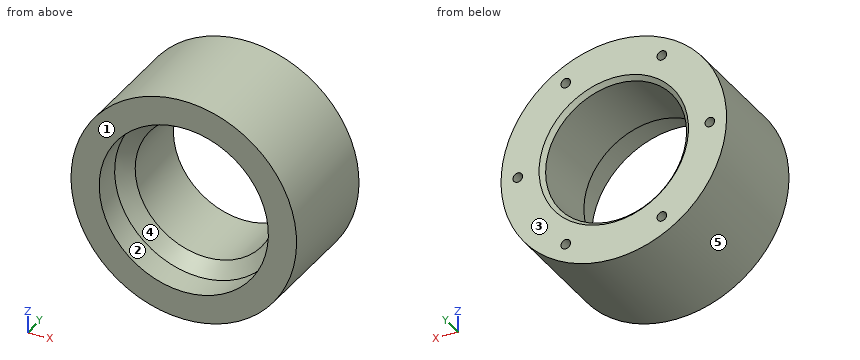
from build123d import *

# Parameters (mm, degrees)
OTW_R_GWINTOWANY_M81_D     = 6.8
OTW_R_GWINTOWANY_M81_DEPTH = 40
OTW_R_GWINTOWANY_M81_TIP   = 2.042926105


with BuildPart() as part:
    # Szkic1 → Obrót1 (revolve)
    with BuildSketch(Plane.XY, mode=Mode.PRIVATE) as obr_t1_sk:
        Polygon((-60, -4.527704194), (-60, 15.472295806), (-60, 76.472295806), (-80, 76.472295806), (-80, -4.527704194), align=None)
        Polygon((-50, 23.863292118), (-50, 73.472295806), (-53, 76.472295806), (-60, 76.472295806), (-60, 15.472295806), align=None)
    revolve(obr_t1_sk.sketch.rotate(Axis((0, 0, 0), (0, 1, 0)), 270), axis=Axis((0, 0, 0), (0, 1, 0)))

    # Otwór gwintowany M81
    with Locations(Plane(origin=(-68.136728334, 76.472295806, 0), x_dir=(0, 0, 1), z_dir=(0, 1, 0))):
        with Locations((0, 0), (-59.008137668, 34.068364167), (-59.008137668, 102.205092501), (0, 136.273456668), (59.008137668, 102.205092501), (59.008137668, 34.068364167)):
            Hole(OTW_R_GWINTOWANY_M81_D / 2, depth=OTW_R_GWINTOWANY_M81_DEPTH)
            with Locations((0, 0, -(OTW_R_GWINTOWANY_M81_DEPTH + OTW_R_GWINTOWANY_M81_TIP / 2))):  # 118° drill point
                Cone(0, OTW_R_GWINTOWANY_M81_D / 2, OTW_R_GWINTOWANY_M81_TIP, mode=Mode.SUBTRACT)


solid = part.part
Here's how the part is built. I have some questions about the finished solid (model axes, mm). Face numbers are marked on the shaded views. A direction names the side the tool comes from. Round coordinates to 2 decimals unless told otherwise and drop trailing zeros. Loops run counter-clockwise (first coordinate to the right, second up) from the corner with the lowest first, then second, coordinate; pieces in that order, holes last.
1. We'd pull the mould along Z, two halves only. Please class the marked faces 3, 4 and 5: +Z half, -Z half, draft (parallel to the pull), parting line (faces both ways), or undercut.
Answer list:
face 3: draft
face 4: undercut
face 5: parting line
2. If we section it at C-C on y = 13.5: Write out the boundary of the cut face in (x, z), plus the area to 3 significant figures.
Answer list:
outline: circle Ø160 at (0, 0); hole circle Ø120 at (0, 0)
area: 8,800 mm2
3. If we section it at B-B on y = 69.5: Write out the boundary of the cut face in (x, z).
Answer list:
outline: circle Ø160 at (0, 0); hole circle Ø6.8 at (-68.14, 0); hole circle Ø100 at (0, 0); hole circle Ø6.8 at (-34.07, -59.01); hole circle Ø6.8 at (-34.07, 59.01); hole circle Ø6.8 at (34.07, -59.01); hole circle Ø6.8 at (34.07, 59.01); hole circle Ø6.8 at (68.14, 0)
4. If I drill on line 1 along X through (y, z) = (52, 0); line 2 along X through (y, z) = (0.5, 0); line 3 along X through (y, z) = (42, 23.5), over which ranges is the centre line in solid material (lowest first)?
Answer list:
line 1: x = -80 to -71.54, -64.74 to -50, 50 to 64.74, 71.54 to 80
line 2: x = -80 to -60, 60 to 80
line 3: x = -76.47 to -44.13, 44.13 to 76.47
5. Which directions (+Z, -Z, +X, -X, +Y, -Y) give clear straight access to the entire face, cutting with the end or side of a thin tool? Please do the marked faces 1 and 2.
Answer list:
face 1: +Z, -Z, +X, -X, -Y
face 2: -Y
6. If we section it at A-A on x = 0: Write out the boundary of the cut face in (y, z), plus the area to 3 significant figures.
Answer list:
outline: (-4.53, -80) - (76.47, -80) - (76.47, -53) - (73.47, -50) - (23.86, -50) - (15.47, -60) - (-4.53, -60) - close; (-4.53, 60) - (15.47, 60) - (23.86, 50) - (73.47, 50) - (76.47, 53) - (76.47, 80) - (-4.53, 80) - close
area: 4,370 mm2
7. If we section it at D-D on z = -66: Write out the boundary of the cut face in (x, y), plus the area to 3 significant figures.
Answer list:
outline: (-45.21, -4.53) - (45.21, -4.53) - (45.21, 76.47) - (-45.21, 76.47) - close
area: 7,320 mm2
8. For P1, Ø8, axis at y = 59, z = 38, coming from the +X side; P2, Ø1, axis at y = 4.5, z = 12.5, coming from the -X side; P3, Ø6, axis at y = 54.5, z = -16, coming from the +X side, each with a flat end and sliding along its axis, tell me the tip position at first contact or that it passes through.
Answer list:
P1: stops at x = 72.42
P2: stops at x = -79.09
P3: stops at x = 78.94
